```python
from build123d import *

# Parameters (mm, degrees)
SKETCH2_W                      = 3
SKETCH2_H                      = 130
BOSS_EXTRUDE1_DEPTH            = 3
SKETCH2_3_W                    = 3
SKETCH2_3_H                    = 130
BOSS_EXTRUDE2_DEPTH            = 30
CUT_EXTRUDE2_DEPTH             = 3
CUT_EXTRUDE3_DEPTH             = 190.092569923
CUT_EXTRUDE3_DEPTH_BACK        = 3
CUT_EXTRUDE4_REACH             = 151.812
CUT_EXTRUDE4_DIRECTION_2_REACH = 151.812
SKETCH9_W                      = 12.4
SKETCH9_H                      = 20
CUT_EXTRUDE5_DEPTH             = 30
CUT_EXTRUDE6_DEPTH             = 11
CUT_EXTRUDE7_DEPTH             = 4.5
CUT_EXTRUDE8_DEPTH             = 17
SKETCH3_W                      = 22.5
SKETCH3_H                      = 22
CUT_EXTRUDE1_DEPTH             = 3
SKETCH10_W                     = 22.5
SKETCH10_H                     = 22
CUT_EXTRUDE9_DEPTH             = 3
CUT_EXTRUDE10_DEPTH            = 190.092569923
FILLET1_R                      = 5
HOLE1_D                        = 3.5
HOLE1_DEPTH                    = 20
HOLE2_D                        = 3.2
HOLE2_DEPTH                    = 4.737087713
HOLE2_CSINK_D                  = 6.4
HOLE2_CSINK_ANGLE              = 90


with BuildPart() as part:
    # Sketch2 → Boss-Extrude1 (new body)
    with BuildSketch(Plane(origin=(0, 0, 0), x_dir=(1, 0, 0), z_dir=(0, 1, 0))):
        Polygon((-3, 130), (-64, 130), (-64, 0), (-9, 0), align=None)
        with Locations((-65.5, 65)):
            Rectangle(SKETCH2_W, SKETCH2_H)
        Polygon((0, 130), (-3, 130), (-9, 0), (0, 0), align=None)
        Polygon((3, 130), (0, 130), (0, 0), (9, 0), align=None)
        Polygon((64, 130), (3, 130), (9, 0), (64, 0), align=None)
        with Locations((65.5, 65)):
            Rectangle(SKETCH2_W, SKETCH2_H)
    extrude(amount=-BOSS_EXTRUDE1_DEPTH)

    # Sketch2<3> → Boss-Extrude2 (add)
    with BuildSketch(Plane(origin=(0, 0, 0), x_dir=(1, 0, 0), z_dir=(0, 1, 0))):
        Polygon((0, 130), (-3, 130), (-9, 0), (0, 0), align=None)
        Polygon((3, 130), (0, 130), (0, 0), (9, 0), align=None)
        with Locations((-65.5, 65)):
            Rectangle(SKETCH2_3_W, SKETCH2_3_H)
        with Locations((65.5, 65)):
            Rectangle(SKETCH2_3_W, SKETCH2_3_H)
    extrude(amount=BOSS_EXTRUDE2_DEPTH)

    # Sketch5 → Cut-Extrude2 (cut)
    with BuildSketch(Plane.ZY.offset(67)):
        Polygon((-130, 30), (-130, 10), (-82.5, 13), (-75, 30), align=None)
    extrude(amount=-CUT_EXTRUDE2_DEPTH, mode=Mode.SUBTRACT)

    # Sketch6 → Cut-Extrude3 (cut, two sides: drawn at the far end of the back side and taken through both)
    with BuildSketch(Plane(origin=(67, 0, 0), x_dir=(0, 0, -1), z_dir=(1, 0, 0)).offset(-CUT_EXTRUDE3_DEPTH_BACK)):
        Polygon((75, 30), (82.5, 13), (130, 10), (130, 30), align=None)
    extrude(amount=CUT_EXTRUDE3_DEPTH + CUT_EXTRUDE3_DEPTH_BACK, mode=Mode.SUBTRACT)

    # Cut-Extrude4: up to this plane
    cut_extrude4_end = Plane(origin=(-8.980869154, 30, -0.414501653), z_dir=(0.9989366098486855, 0, 0.04610476660840086))
    # Sketch7 → Cut-Extrude4 (cut, up to the surface)
    with BuildSketch(Plane(origin=(1.5, 0, -0.187149168), x_dir=(0, 0, -1), z_dir=(1, 0, 0)), mode=Mode.PRIVATE) as cut_extrude4_sk1:
        Polygon((129.812850832, 7), (74.312850832, 10), (57.312850832, 30), (129.812850832, 30), align=None)
    cut_extrude4_tool1 = split(extrude(cut_extrude4_sk1.sketch, amount=-CUT_EXTRUDE4_REACH, mode=Mode.PRIVATE), bisect_by=cut_extrude4_end, keep=Keep.BOTH, mode=Mode.PRIVATE)
    add(cut_extrude4_tool1.solids().sort_by_distance((1.5, 19.743933, -98.647747))[0], mode=Mode.SUBTRACT)

    # Cut-Extrude4 direction 2: up to this plane
    cut_extrude4_direction_2_end = Plane(origin=(8.980869154, 30, -0.414501653), z_dir=(0.9989366098486855, 0, -0.04610476660840086))
    # Sketch7 → Cut-Extrude4 direction 2 (cut, up to the surface)
    with BuildSketch(Plane(origin=(1.5, 0, -0.187149168), x_dir=(0, 0, -1), z_dir=(1, 0, 0)), mode=Mode.PRIVATE) as cut_extrude4_direction_2_sk1:
        Polygon((129.812850832, 7), (74.312850832, 10), (57.312850832, 30), (129.812850832, 30), align=None)
    cut_extrude4_direction_2_tool1 = split(extrude(cut_extrude4_direction_2_sk1.sketch, amount=CUT_EXTRUDE4_DIRECTION_2_REACH, mode=Mode.PRIVATE), bisect_by=cut_extrude4_direction_2_end, keep=Keep.BOTH, mode=Mode.PRIVATE)
    add(cut_extrude4_direction_2_tool1.solids().sort_by_distance((1.5, 19.743933, -98.647747))[0], mode=Mode.SUBTRACT)

    # Sketch9 → Cut-Extrude5 (cut)
    with BuildSketch(Plane.XY):
        with Locations((0, 20)):
            Rectangle(SKETCH9_W, SKETCH9_H)
    extrude(amount=-CUT_EXTRUDE5_DEPTH, mode=Mode.SUBTRACT)

    # Sketch9<3> → Cut-Extrude6 (cut)
    with BuildSketch(Plane.XY):
        with BuildLine():
            Line((0, 10), (-6.2, 10))
            Line((-6.2, 10), (-6.2, 4.9))
            Line((-6.2, 4.9), (0, 4.9))
            Line((0, 4.9), (0, 6.2))
            ThreePointArc((0, 6.2), (-1.25, 7.45), (0, 8.7))
            Line((0, 8.7), (0, 10))
        make_face()
        with BuildLine():
            Line((6.2, 4.9), (6.2, 10))
            Line((6.2, 10), (0, 10))
            Line((0, 10), (0, 8.7))
            ThreePointArc((0, 8.7), (0.883883476, 8.333883476), (1.25, 7.45))
            ThreePointArc((1.25, 7.45), (0.883883476, 6.566116524), (0, 6.2))
            Line((0, 6.2), (0, 4.9))
            Line((0, 4.9), (6.2, 4.9))
        make_face()
    extrude(amount=-CUT_EXTRUDE6_DEPTH, mode=Mode.SUBTRACT)

    # Sketch9<4> → Cut-Extrude7 (cut)
    with BuildSketch(Plane.XY):
        Polygon((-6.2, 10), (-6.2, 30), (-9, 30), (-9, 0), (9, 0), (9, 30), (6.2, 30), (6.2, 10), (6.2, 4.9), (-6.2, 4.9), align=None)
        Polygon((9, 0), (-9, 0), (-64, 0), (-64, -3), (64, -3), (64, 0), align=None)
    extrude(amount=-CUT_EXTRUDE7_DEPTH, mode=Mode.SUBTRACT)

    # Sketch9<5> → Cut-Extrude8 (cut)
    with BuildSketch(Plane.XY):
        with BuildLine():
            ThreePointArc((1.25, 7.45), (0.883883476, 8.333883476), (0, 8.7))
            Line((0, 8.7), (0, 6.2))
            ThreePointArc((0, 6.2), (0.883883476, 6.566116524), (1.25, 7.45))
        make_face()
        with BuildLine():
            Line((0, 6.2), (0, 8.7))
            ThreePointArc((0, 8.7), (-1.25, 7.45), (0, 6.2))
        make_face()
    extrude(amount=-CUT_EXTRUDE8_DEPTH, mode=Mode.SUBTRACT)

    # Sketch3 → Cut-Extrude1 (cut)
    with BuildSketch(Plane.ZY.offset(67)):
        Polygon((-50.727683193, 4.5), (-78.052542275, 4.5), (-68.346659922, 26.5), (-41.02180084, 26.5), align=None)
        with Locations((-18.75, 15.5)):
            Rectangle(SKETCH3_W, SKETCH3_H)
        Polygon((-30, 4.5), (-30, 26.5), (-39.705882353, 4.5), align=None)
    extrude(amount=-CUT_EXTRUDE1_DEPTH, mode=Mode.SUBTRACT)

    # Sketch10 → Cut-Extrude9 (cut)
    with BuildSketch(Plane(origin=(67, 0, 0), x_dir=(0, 0, -1), z_dir=(1, 0, 0))):
        with Locations((18.75, 15.5)):
            Rectangle(SKETCH10_W, SKETCH10_H)
        Polygon((30, 4.5), (30, 26.5), (39.705882353, 4.5), align=None)
        Polygon((50.727683193, 4.5), (78.052542275, 4.5), (68.346659922, 26.5), (41.02180084, 26.5), align=None)
    extrude(amount=-CUT_EXTRUDE9_DEPTH, mode=Mode.SUBTRACT)

    # Sketch11 → Cut-Extrude10 (cut, through all)
    with BuildSketch(Plane.ZY.offset(67)):
        Polygon((0, -3), (-3.759875074, 30), (0, 30), align=None)
    extrude(amount=-CUT_EXTRUDE10_DEPTH, mode=Mode.SUBTRACT)

    # Fillet1
    fillet1_edges = [part.edges().sort_by_distance(p)[0] for p in [
        (-65.5, 30, -75),
        (-65.5, 10, -130),
        (-65.5, 13, -82.5),
        (65.5, 30, -75),
        (65.5, 13, -82.5),
        (65.5, 10, -130),
        (0, 10, -74.5),
        (0, 30, -57.5),
        (0, 7, -130),
    ]]
    fillet(fillet1_edges, radius=FILLET1_R)

    # Hole1
    with Locations(Plane(origin=(0, 30, -47.593898813), x_dir=(0, 0, 1), z_dir=(0, 1, 0))):
        with Locations((0, 0), (10, 0)):
            Hole(HOLE1_D / 2, depth=HOLE1_DEPTH)

    # Hole2
    with Locations(Plane(origin=(-51, 0, -120), x_dir=(0, 0, 1), z_dir=(0, 1, 0))):
        with Locations((0, 0), (0, 105), (95.5, 105), (95.5, 0)):
            CounterSinkHole(HOLE2_D / 2, HOLE2_CSINK_D / 2, depth=HOLE2_DEPTH, counter_sink_angle=HOLE2_CSINK_ANGLE)


solid = part.part
```
Model file for the job. Use its own axes, mm. A direction names the side the tool comes from. Give positions to 0.01 mm unless a question says otherwise; leave off trailing zeros. Write each loop counter-clockwise with the first axis right and the second up, starting at its lowest first coordinate (ties: lowest second). Pieces come first, ordered by that corner, then holes. Notation, with made-up numbers: (38, 45.5) -> (58, 45.5) arc R20 ccw to (58, 60.5) -> close; hole circle Ø4 at (40.25, 21.5). An arc over 180 degrees is marked (long way). Use CSV: the item, a comma, the result in double quotes. Start each with the question number.
1) Cut at D-D on z = -97. List the corners of the cut face in (x, y).
2) Cut at B-B on y = 24. Count the separate pieces of the cut face and the enclosed holes in it, plus the area to 3 significant figures.
3) Drill centre lines: L1, parallel to Z at x = 54, y = -2; L2, parallel to X at y = -2.2, z = -24.5; L3, parallel to X at y = 4, z = -88.5. Where is each one in solid material? Low to high.
4) Cut at C-C on z = -120. List the corners of the cut face in (x, y).
5) Cut at A-A on x = 54. List the corners of the cut face in (y, z).
6) Pin check, flat tips, straight feed: P1, Ø4.5, axis at x = 0, z = -37.59, coming from the +Y side; P2, Ø3.5, axis at x = -1, y = 21.5, coming from the +Z side; P3, Ø10, axis at x = -16, z = -64.5, coming from the +Y side; P4, Ø1.5, axis at y = 22, z = -52.5, coming from the +X side. Stop position of each tip, or through.
7) Two-plate mould, pull along Z, no slides. Class faces 1 (the flat face through (0, -1, -4.5)), 2 (the flat face through (-65.52, 15.65, -45.81)), 3 (the flat face through (-66, 30, -38)): released by +Z, released by -Z, zero draft, split by the parting line, or undercut.
8) Tool access for faces 4 (the flat face through (-66, 26.5, -19)), 5 (the cylindrical face through (0.079, 10.384, -74.722)), 6 (the flat face through (65.521, 15.346, -73.268)): list every direction of +Z, -Z, +X, -X, +Y, -Y with a clear straight run to the whole face (end or side of a thin tool).
Final values:
1,outline,"(-67, -3) -> (67, -3) -> (67, 12.08) -> (64, 12.08) -> (64, 0) -> (4.52, 0) -> (4.52, 8.78) -> (-4.52, 8.78) -> (-4.52, 0) -> (-64, 0) -> (-64, 12.08) -> (-67, 12.08) -> close"
2,separate pieces,"7"
2,enclosed holes,"2"
2,area,"672 mm2"
3,L1,"z = -130 to -121.6, -118.4 to -26.1, -22.9 to -4.5"
3,L2,"x = -67 to -52.6, -49.4 to 52.4, 55.6 to 67"
3,L3,"x = -67 to -64, -4.92 to 4.92, 64 to 67"
4,outline,"(-67, -3) -> (-52.6, -3) -> (-52.6, -1.6) -> (-54.2, 0) -> (-64, 0) -> (-64, 10.63) -> (-67, 10.63) -> close; (-49.4, -3) -> (52.4, -3) -> (52.4, -1.6) -> (50.8, 0) -> (3.46, 0) -> (3.46, 7.54) -> (-3.46, 7.54) -> (-3.46, 0) -> (-47.8, 0) -> (-49.4, -1.6) -> close; (55.6, -3) -> (67, -3) -> (67, 10.63) -> (64, 10.63) -> (64, 0) -> (57.2, 0) -> (55.6, -1.6) -> close"
5,outline,"(-3, -130) -> (0, -130) -> (0, -123.2) -> (-1.6, -121.6) -> (-3, -121.6) -> close; (-3, -118.4) -> (-1.6, -118.4) -> (0, -116.8) -> (0, -27.7) -> (-1.6, -26.1) -> (-3, -26.1) -> close; (-3, -22.9) -> (-1.6, -22.9) -> (0, -21.3) -> (0, -4.5) -> (-3, -4.5) -> close"
6,P1,"stops at y = 30"
6,P2,"stops at z = -30"
6,P3,"stops at y = 0"
6,P4,"stops at x = 6.61"
7,face 1,"released by +Z"
7,face 2,"undercut"
7,face 3,"zero draft"
8,face 4,"-X"
8,face 5,"-Z, +Y"
8,face 6,"+X"
